Can you work these out from the model? Positions are in its coordinate system, mm. Round coordinates to 2 decimals unless told otherwise and drop trailing zeros. Order: outer loops, then holes, each group sorted by start corner. A loop starts at its lowest first (then second) coordinate and runs counter-clockwise, first axis right, second up. Notation, with made-up numbers: M 49.5,2 L 65.5,2 A12 cw 65.5,12 Z; hole C 51,46.5 d7. An arc over 180 degrees is marked long. One line per question, with ' | ' between items.
```python
from build123d import *

# Parameters (mm, degrees)
F0_W     = 100
F0_H     = 200
F0_R     = 7.5
F0_R_2   = 15
F0_R_3   = 22.5
F1_DEPTH = 25
F2_SIZE  = 5
F3_DEPTH = 25
F4_SIZE  = 5
F5_SIZE  = 3


# Not quite as in the source:
# - a feature names something its author has since deleted; it is built from what else it names


with BuildPart() as f1:
    # F0 (on Right) → F1 (new body)
    with BuildSketch(Plane.YZ):
        Rectangle(F0_W, F0_H)
        with Locations((0, -75)):
            Circle(F0_R, mode=Mode.SUBTRACT)
        with Locations((0, -25)):
            Circle(F0_R_2, mode=Mode.SUBTRACT)
        with Locations((0, 50)):
            Circle(F0_R_3, mode=Mode.SUBTRACT)
    extrude(amount=F1_DEPTH)

    # F2
    f2_edges = [f1.edges().sort_by_distance(p)[0] for p in [
        (25, 50, 0),
        (0, 50, 0),
        (12.5, 22.5, 50),
        (0, -22.5, 50),
        (25, -22.5, 50),
        (12.5, 7.5, -75),
        (0, -7.5, -75),
        (25, -7.5, -75),
        (0, -50, 0),
        (25, -50, 0),
        (25, 0, -100),
        (0, 0, -100),
        (0, 0, 100),
        (25, 0, 100),
    ]]
    chamfer(f2_edges, length=F2_SIZE)

    # F0 (on Right) → F3 (join)
    with BuildSketch(Plane.YZ):
        Rectangle(F0_W, F0_H)
        with Locations((0, -75)):
            Circle(F0_R, mode=Mode.SUBTRACT)
        with Locations((0, -25)):
            Circle(F0_R_2, mode=Mode.SUBTRACT)
        with Locations((0, 50)):
            Circle(F0_R_3, mode=Mode.SUBTRACT)
    extrude(amount=F3_DEPTH)

    # F4
    f4_edges = [f1.edges().sort_by_distance(p)[0] for p in [
        (25, 0, 100),
        (25, -50, 0),
        (25, 0, -100),
        (25, 50, 0),
        (0, -50, 0),
        (0, 0, 100),
        (0, 50, 0),
        (0, 0, -100),
    ]]
    chamfer(f4_edges, length=F4_SIZE)

    # F5
    f5_edges = [f1.edges().sort_by_distance(p)[0] for p in [
        (0, -22.5, 50),
        (12.5, 22.5, 50),
        (25, -22.5, 50),
        (12.5, 15, -25),
        (0, -15, -25),
        (25, -15, -25),
        (0, -7.5, -75),
        (12.5, 7.5, -75),
        (25, -7.5, -75),
    ]]
    chamfer(f5_edges, length=F5_SIZE)


solid = f1.part
```
(1) Thinking about a two-plate mould opening in Z: for faces 1 (the flat face through (23, 47, -1)), 2 (the cylindrical face through (12.367, -3.252, -39.643)), 3 (the flat face through (2, -1, -97)), which applies, released by +Z, released by -Z, zero draft, split by the parting line, or undercut?
Final values:
face 1: zero draft | face 2: undercut | face 3: released by -Z
(2) If we section it at A-A on z = -75: Please give me the cut outline in (x, y), plus the area to 3 significant figures.
Final values:
outline: M 0,-45 L 5,-50 L 20,-50 L 25,-45 L 25,-10.5 L 22,-7.5 L 3,-7.5 L 0,-10.5 Z; M 0,10.5 L 3,7.5 L 22,7.5 L 25,10.5 L 25,45 L 20,50 L 5,50 L 0,45 Z | area: 2,060 mm^2
(3) If we section it at B-B on y = 0: State how many separate pieces and enclosed holes the cut face has, plus the area to 3 significant figures.
Final values:
separate pieces: 4 | enclosed holes: 0 | area: 2,650 mm^2
(4) If we section it at C-C on x = 7.25: Please give me the cut outline in (y, z), plus the area to 3 significant figures.
Final values:
outline: M -50,-100 L 50,-100 L 50,100 L -50,100 Z; hole C 0,50 d45; hole C 0,-25 d30; hole C 0,-75 d15 | area: 17,500 mm^2
(5) Please list where these lines run through material, in increasing order: probe 1 along Z at (x, y) = (9.5, 0); probe 2 along Z at (x, y) = (11, 2); probe 3 along Z at (x, y) = (5.5, 13). Write a range as [from, to].
Final values:
probe 1: [-100, -82.5], [-67.5, -40], [-10, 27.5], [72.5, 100] | probe 2: [-100, -82.23], [-67.77, -39.87], [-10.13, 27.59], [72.41, 100] | probe 3: [-100, -32.48], [-17.52, 31.64], [68.36, 100]
(6) Will this pin go through, and if not, where does the flat tip stop? pin 1 Ø17 at (y, z) = (0, -75) entering from -X.
Final values:
pin 1: x = 2
(7) If we section it at D-D on z = 81.5: Please give me the cut outline in (x, y).
Final values:
outline: M 0,-45 L 5,-50 L 20,-50 L 25,-45 L 25,45 L 20,50 L 5,50 L 0,45 Z
